Work out the finished part from the listing and answer in its coordinate system (mm). A direction names the side the tool comes from. Give positions to 0.01 mm unless a question says otherwise; leave off trailing zeros. Loops run counter-clockwise (first coordinate to the right, second up) from the corner with the lowest first, then second, coordinate; pieces in that order, holes last.
```python
from build123d import *

# Parameters (mm, degrees)
F1_DEPTH = 7
F2_DEPTH = 6
F3_R     = 2
F4_DEPTH = 25
F6_DEPTH = 25


# Not quite as in the source:
# - a pattern or mirror of a feature is missing from the dataset's text; its kind, count and spacing are read off the source's solid


with BuildPart() as f1:
    # F0 (on Front) → F1 (new body, symmetric)
    with BuildSketch(Plane.XZ):
        with BuildLine():
            Line((129.5, 0), (174.5, 0))
            ThreePointArc((174.5, 0), (174.2671322418, 9.0120264206), (173.5691504848, 18))
            ThreePointArc((173.5691504848, 18), (0, 174.5), (-173.5691504848, 18))
            ThreePointArc((-173.5691504848, 18), (-174.2671322418, 9.0120264206), (-174.5, 0))
            Line((-174.5, 0), (-129.5, 0))
            ThreePointArc((-129.5, 0), (0, 129.5), (129.5, 0))
        make_face()
        with BuildLine():
            ThreePointArc((173.5691504848, 18), (174.2671322418, 9.0120264206), (174.5, 0))
            Line((174.5, 0), (194.5, 0))
            Line((194.5, 0), (194.5, 18))
            Line((194.5, 18), (173.5691504848, 18))
        make_face()
        with BuildLine():
            ThreePointArc((-174.5, 0), (-174.2671322418, 9.0120264206), (-173.5691504848, 18))
            Line((-173.5691504848, 18), (-194.5, 18))
            Line((-194.5, 18), (-194.5, 0))
            Line((-194.5, 0), (-174.5, 0))
        make_face()
    extrude(amount=F1_DEPTH, both=True)

    # F0 (on Front) → F2 (join, symmetric)
    with BuildSketch(Plane.XZ):
        with BuildLine():
            Line((129.5, 0), (174.5, 0))
            ThreePointArc((174.5, 0), (174.2671322418, 9.0120264206), (173.5691504848, 18))
            ThreePointArc((173.5691504848, 18), (0, 174.5), (-173.5691504848, 18))
            ThreePointArc((-173.5691504848, 18), (-174.2671322418, 9.0120264206), (-174.5, 0))
            Line((-174.5, 0), (-129.5, 0))
            ThreePointArc((-129.5, 0), (0, 129.5), (129.5, 0))
        make_face()
        with BuildLine():
            ThreePointArc((173.5691504848, 18), (174.2671322418, 9.0120264206), (174.5, 0))
            Line((174.5, 0), (194.5, 0))
            Line((194.5, 0), (194.5, 18))
            Line((194.5, 18), (173.5691504848, 18))
        make_face()
        with BuildLine():
            ThreePointArc((-174.5, 0), (-174.2671322418, 9.0120264206), (-173.5691504848, 18))
            Line((-173.5691504848, 18), (-194.5, 18))
            Line((-194.5, 18), (-194.5, 0))
            Line((-194.5, 0), (-174.5, 0))
        make_face()
    extrude(amount=F2_DEPTH, both=True)

    # F3 (on face) → F4 (cut)
    with BuildSketch(Plane.XZ.offset(7)):
        with Locations((185.5, 9)):
            Circle(F3_R)
    f4 = extrude(amount=-F4_DEPTH, mode=Mode.SUBTRACT)

    # F4_copies: F4 across plane
    add(f4.mirror(Plane(origin=(0, 0, 0), x_dir=(0, 0, -1), z_dir=(-1, 0, 0))), mode=Mode.SUBTRACT)

    # F5 (on face) → F6 (cut)
    with BuildSketch(Plane.XY.offset(18)):
        with BuildLine():
            Line((194.5, 3), (178.5, 3))
            ThreePointArc((178.5, 3), (175.5, 0), (178.5, -3))
            Line((178.5, -3), (194.5, -3))
            Line((194.5, -3), (194.5, 3))
        make_face()
    f6 = extrude(amount=-F6_DEPTH, mode=Mode.SUBTRACT)

    # F6_copies: F6 across plane
    add(f6.mirror(Plane(origin=(0, 0, 0), x_dir=(0, 0, -1), z_dir=(-1, 0, 0))), mode=Mode.SUBTRACT)


solid = f1.part
```
Q1. Section C-C on x = 0 is taken. Give the vertices of the cut face in (y, z), plus the area to 3 significant figures.
Q2. Section B-B on y = 0 is taken. Give the vertices of the cut face in (x, z).
Q3. Given pin 1 (4.5 mm diameter, centred on x = 185.5, z = 9, fed in from +Y); pin 2 (4 mm diameter, centred on x = 180, y = 2.5, fed in from +Z); pin 3 (3 mm diameter, centred on x = -185.5, z = 9, fed in from -Y); pin 4 (4 mm diameter, centred on x = 87, y = 3, fed in from +Z), each flat-ended and moving along its own axis, determine where each tip first touches the part or whether it passes through.
Q4. Consider line 1 along Z through (x, y) = (-185.5, -4.1); line 2 along Z through (x, y) = (3.5, 2.5); line 3 along X through (y, z) = (0.5, 65). Determine where each line is inside the solid, lowest interval first.
Q5. Section A-A on z = 31 is taken. Give the vertices of the cut face in (x, y).
Q6. Which of the six approach directions +Z, -Z, +X, -X, +Y, -Y give full straight-line access (tool end or side, diameter ignored) to faces 1 (the face through (-188, 3, 9)), 2 (the face through (184.2, -3.2, 18)), 3 (the face through (188, -3, 9)), 4 (the face through (162, 0, 0))?
Q7. Section D-D on z = 114.5 is taken. Give the vertices of the cut face in (x, y), plus the area to 3 significant figures.
Q8. Determine the mould class of faces 5 (the face through (188, 3, 9)), 6 (the face through (-183.9, -3.2, 18)), 7 (the face through (-1, -7, 133)) for opening direction Y: +Y half, -Y half, draft (parallel to the pull), parting line (faces both ways), or undercut.
Check result:
1. outline: (-7, 129.5) - (7, 129.5) - (7, 174.5) - (-7, 174.5) - close
1. area: 630 mm2
2. outline: (-175.5, 0) - (-129.5, 0) arc R129.5 cw to (129.5, 0) - (175.5, 0) - (175.5, 18) - (173.57, 18) arc R174.5 ccw to (-173.57, 18) - (-175.5, 18) - close
3. pin 1: stops at y = 7
3. pin 2: stops at z = 18
3. pin 3: passes through
3. pin 4: stops at z = 152.4
4. line 1: z = 0 to 7, 11 to 18
4. line 2: z = 129.45 to 174.46
4. line 3: x = -161.94 to -112.01, 112.01 to 161.94
5. outline: (-171.72, -7) - (-125.73, -7) - (-125.73, 7) - (-171.72, 7) - close; (125.73, -7) - (171.72, -7) - (171.72, 7) - (125.73, 7) - close
6. face 1: +Z, -Z, -X
6. face 2: +Z, +X, +Y, -Y
6. face 3: +Z, -Z, +X
6. face 4: -Z, +X, -X, +Y, -Y
7. outline: (-131.68, -7) - (-60.5, -7) - (-60.5, 7) - (-131.68, 7) - close; (60.5, -7) - (131.68, -7) - (131.68, 7) - (60.5, 7) - close
7. area: 1,990 mm2
8. face 5: undercut
8. face 6: draft
8. face 7: -Y half
